```python
from build123d import *

# Parameters (mm, degrees)
CUT_EXTRUDE1_START = -5.461
CUT_EXTRUDE1_DEPTH = 5.461
CHAMFER1_SIZE      = 0.254


with BuildPart() as part:
    # Sketch3 → Revolve1 (revolve)
    with BuildSketch(Plane.XY):
        with BuildLine():
            Line((0, 12.192), (-1.905, 12.192))
            Line((-1.905, 12.192), (-1.905, 3.002683966))
            ThreePointArc((-1.905, 3.002683966), (-2.985336827, 1.932071435), (-3.519527241, 0.508))
            Line((-3.519527241, 0.508), (-2.639645431, 0.508))
            Line((-2.639645431, 0.508), (-2.199704526, 1.27))
            ThreePointArc((-2.199704526, 1.27), (-1.796051224, 1.796051224), (-1.27, 2.199704526))
            Line((-1.27, 2.199704526), (0, 2.932939367))
            Line((0, 2.932939367), (0, 12.192))
        make_face()
    revolve(axis=Axis((0, 12.192, 0), (0, -1, 0)))

    # Sketch4 → Cut-Extrude1 (cut)
    with BuildSketch(Plane(origin=(0, 12.192, 0), x_dir=(1, 0, 0), z_dir=(0, 1, 0)).offset(CUT_EXTRUDE1_START)):
        with BuildLine():
            Line((1.5875, 1.053028371), (1.5875, -1.053028371))
            ThreePointArc((1.5875, -1.053028371), (1.905, 0), (1.5875, 1.053028371))
        make_face()
        with BuildLine():
            Line((0.508, 1.053028371), (1.5875, 1.053028371))
            ThreePointArc((1.5875, 1.053028371), (1.118502631, 1.542069021), (0.508, 1.836017701))
            Line((0.508, 1.836017701), (0.508, 1.053028371))
        make_face()
        with BuildLine():
            ThreePointArc((-1.5875, 1.053028371), (-1.905, 0), (-1.5875, -1.053028371))
            Line((-1.5875, -1.053028371), (-1.5875, 1.053028371))
        make_face()
        with BuildLine():
            Line((-0.508, 1.836017701), (0.508, 1.836017701))
            ThreePointArc((0.508, 1.836017701), (0, 1.905), (-0.508, 1.836017701))
        make_face()
        with BuildLine():
            ThreePointArc((-0.508, 1.836017701), (-1.118502631, 1.542069021), (-1.5875, 1.053028371))
            Line((-1.5875, 1.053028371), (-0.508, 1.053028371))
            Line((-0.508, 1.053028371), (-0.508, 1.836017701))
        make_face()
    extrude(amount=CUT_EXTRUDE1_DEPTH, mode=Mode.SUBTRACT)

    # Chamfer1
    # the kernel refuses this chamfer: 0.254, 0.224262667 mm, written as the material it takes off along each edge
    with BuildSketch(Plane(origin=(0, 0.508, 0), x_dir=(-1, 0, 0), z_dir=(0, 0, 1))) as chamfer1_piece_1:
        with BuildLine():
            Line((3.519527241 - CHAMFER1_SIZE, 0), (3.481518689, -0.215991448))
            ThreePointArc((3.481518689, -0.215991448), (3.501682417, -0.111157692), (3.519527241, 0))
            Line((3.519527241, 0), (3.519527241 - CHAMFER1_SIZE, 0))
        make_face()
    revolve(axis=Axis((0, 0.508, 0), (0, -1, 0)), mode=Mode.SUBTRACT)


solid = part.part
```
Here's how the part is built. I have some questions about the finished solid (model axes, mm). A direction names the side the tool comes from. Round coordinates to 2 decimals unless told otherwise and drop trailing zeros. Order: outer loops, then holes, each group sorted by start corner. A loop starts at its lowest first (then second) coordinate and runs counter-clockwise, first axis right, second up. Notation, with made-up numbers: M -34,-11.75 L 9,-11.75 A22 ccw 9,17.25 Z; hole C -5,8.25 d9. An arc over 180 degrees is marked long. Answer in a Markdown table with one row per item.
Item 1: For faces 1 (the face through (0.41, 6.51, 1.86)), 2 (the face through (-1.588, 9, 0)), 3 (the face through (0, 9, -1.836)), 4 (the face through (-1, 9, -1.053)), which set-ups out of +Z, -Z, +X, -X, +Y, -Y let a thin tool reach every point of the face, with its end or its side?
A:
| item | result |
|---|---|
| face 1 | +Y |
| face 2 | +Z, -Z, -X, +Y |
| face 3 | -Z, +X, -X, +Y |
| face 4 | -Z, -X, +Y |
Item 2: Imagine slicing it at B-B, the plane y = 5.75. Write out the boundary of the cut face in (x, z) (3 decimals).
A:
| item | result |
|---|---|
| outline | C 0,0 d3.81 |
Item 3: If I drill on L1, parallel to X at y = 3.5, z = 0 (3 decimals); L2, parallel to X at y = 8, z = 0.25; L3, parallel to Y at x = 0.25, z = 3, over which ranges is the centre line in solid material (lowest first)? Write a range as from..to.
A:
| item | result |
|---|---|
| L1 | x = -1.905..1.905 |
| L2 | x = -1.59..1.59 |
| L3 | y = 0.51..1.89 |
Item 4: Thinking about a two-plate mould opening in Z: for faces 5 (the face through (0.161, 2.816, 0.123)), 6 (the face through (1, 9, -1.053)), 7 (the face through (1.588, 9, 0)), which applies, +Z half, -Z half, draft (parallel to the pull), parting line (faces both ways), or undercut?
A:
| item | result |
|---|---|
| face 5 | undercut |
| face 6 | -Z half |
| face 7 | draft |
Item 5: Imagine slicing it at A-A, the plane y = 8.5. Write out the boundary of the cut face in (x, z) (1 decimal), and give its area (3 significant figures).
A:
| item | result |
|---|---|
| outline | M -1.6,-1.1 L -0.5,-1.1 L -0.5,-1.8 L 0.5,-1.8 L 0.5,-1.1 L 1.6,-1.1 L 1.6,1.1 A1.9 ccw -1.6,1.1 Z |
| area | 9.39 mm2 |
Item 6: I'm going to push flat-ended pins straight in: pin 1 (4 mm diameter, centred on x = 0, y = 4.5, fed in from -Z); pin 2 (0.6 mm diameter, centred on y = 9.5, z = 0.5, fed in from -X); pin 3 (0.6 mm diameter, centred on y = 10, z = 0, fed in from +X). Where does each tip first touch, or does it pass through?
A:
| item | result |
|---|---|
| pin 1 | stops at z = -2.53 |
| pin 2 | stops at x = -1.59 |
| pin 3 | stops at x = 1.59 |
